Here's how the part is built. I have some questions about the finished solid (model axes, mm). A direction names the side the tool comes from. Coordinates: 2 decimals unless noted, no trailing zeros. Write each loop counter-clockwise with the first axis right and the second up, starting at its lowest first coordinate (ties: lowest second). Pieces come first, ordered by that corner, then holes. Notation, with made-up numbers: (13.25, -3) -> (50.25, -3) arc R27 ccw to (50.25, 34) -> close; hole circle Ø5 at (40, 31.25). An arc over 180 degrees is marked (long way). Use a Markdown table: item, result. Add a question column.
```python
from build123d import *

# Parameters (mm, degrees)
BOSS_EXTRUDE1_DEPTH      = 18
REVOLVE1_ANGLE           = 155
REVOLVE1_OTHER_WAY_ANGLE = 135
CHAMFER1_SIZE            = 2


with BuildPart() as part:
    # Sketch1 → Boss-Extrude1 (new body)
    with BuildSketch(Plane.XY):
        with BuildLine():
            ThreePointArc((26.284248015, 72.215377907), (13.344862454, -75.682475819), (-49.398227804, 58.870515454))
            ThreePointArc((-49.398227804, 58.870515454), (-48.984779038, 59.542460442), (-49.056117508, 60.328183531))
            ThreePointArc((-49.056117508, 60.328183531), (-49.916101751, 61.045004286), (-51.005196829, 60.785626561))
            ThreePointArc((-51.005196829, 60.785626561), (13.778982898, -78.144495202), (27.139298373, 74.564609459))
            ThreePointArc((27.139298373, 74.564609459), (22.507336673, 84.497883381), (32.440610594, 89.129845082))
            ThreePointArc((32.440610594, 89.129845082), (32.488426827, 89.113527981), (32.536863386, 89.099156495))
            ThreePointArc((32.536863386, 89.099156495), (34.05906865, 89.924751911), (33.295660953, 91.479076634))
            ThreePointArc((33.295660953, 91.479076634), (20.158105121, 85.35293374), (26.284248015, 72.215377907))
        make_face()
    extrude(amount=BOSS_EXTRUDE1_DEPTH)

    # Sketch2 → Revolve1 (revolve)
    with BuildSketch(Plane(origin=(0, 0, 0), x_dir=(0, 0, -1), z_dir=(1, 0, 0))):
        Polygon((-14, -74.85), (-16, -76.85), (-2, -76.85), (-4, -74.85), align=None)
    revolve(axis=Axis((0, 0, 0), (0, 0, 1)), revolution_arc=REVOLVE1_ANGLE)

    # Sketch2 → Revolve1 other way (revolve)
    with BuildSketch(Plane(origin=(0, 0, 0), x_dir=(0, 0, -1), z_dir=(1, 0, 0))):
        Polygon((-14, -74.85), (-16, -76.85), (-2, -76.85), (-4, -74.85), align=None)
    revolve(axis=Axis((0, 0, 0), (0, 0, -1)), revolution_arc=REVOLVE1_OTHER_WAY_ANGLE)

    # Chamfer1
    # the kernel refuses this chamfer: 2 mm, written as the material it takes off along each edge
    with BuildSketch(Plane(origin=(31.632976891, 67.83713786, -1.214315162), x_dir=(0.9005003860175051, -0.4348552112856927, 0), z_dir=(0, 0, 1))) as chamfer1_piece_1_section:
        with BuildLine():
            Line((2.027650031, 0), (-CHAMFER1_SIZE * 0.0135447563861, CHAMFER1_SIZE * 0.99990826558))
            Line((-CHAMFER1_SIZE * 0.0135447563861, CHAMFER1_SIZE * 0.99990826558), (0, 0))
            ThreePointArc((0, 0), (1.042503113, 0.006860827), (2.027650031, 0))
        make_face()
    chamfer1_piece_1 = extrude(amount=20.428630325, mode=Mode.PRIVATE)
    chamfer1_piece_1 = chamfer1_piece_1 & Plane(origin=(0, 0, -1.214315162), x_dir=(0.3420201433256637, 0.9396926207859103, 0), z_dir=(0, 0, -1)) * Cylinder(76.85, 49, mode=Mode.PRIVATE)
    add(chamfer1_piece_1, mode=Mode.SUBTRACT)
    with BuildSketch(Plane(origin=(-52.926942572, 52.926942572, -1.214315162), x_dir=(-0.6974643260656699, -0.7166195042459848, 0), z_dir=(0, 0, 1))) as chamfer1_piece_2_section:
        with BuildLine():
            Line((2.027650031, 0), (-CHAMFER1_SIZE * 0.0135447563861, -CHAMFER1_SIZE * 0.99990826558))
            Line((-CHAMFER1_SIZE * 0.0135447563861, -CHAMFER1_SIZE * 0.99990826558), (0, 0))
            ThreePointArc((0, 0), (1.042503113, -0.006860827), (2.027650031, 0))
        make_face()
    chamfer1_piece_2 = extrude(amount=20.428630325, mode=Mode.PRIVATE)
    chamfer1_piece_2 = chamfer1_piece_2 & Plane(origin=(0, 0, -1.214315162), x_dir=(0.3420201433256637, 0.9396926207859103, 0), z_dir=(0, 0, -1)) * Cylinder(76.85, 49, mode=Mode.PRIVATE)
    add(chamfer1_piece_2, mode=Mode.SUBTRACT)


solid = part.part
```
Q1. Suppose I cut it at C-C, the plane z = 8.5. Write out the boundary of the cut face in (x, y), and give its area (3 significant figures).
Q2. Please list where these lines run through material, in increasing order: line 1 (Y direction, x = 28.5, z = 3.25); line 2 (X direction, y = 0, z = 8); line 3 (Y direction, x = 0, z = 8.25).
Q3. Suppose I cut it at A-A, the plane y = 0. Write out the boundary of the cut face in (x, z).
Q4. Will these pins go through, and if not, where does the flat tip stop? pin 1 (8 mm diameter, centred on y = 67.5, z = 5.5, fed in from +X); pin 2 (5 mm diameter, centred on y = -57.5, z = 7.5, fed in from +X); pin 3 (5 mm diameter, centred on x = 2.5, z = 7, fed in from +Y).
Q5. Which directions (+Z, -Z, +X, -X, +Y, -Y) give clear straight access to the entire face, cutting with the end or side of a thin tool? Please do faces 1 (the flat face through (-53, -57, 18)), 2 (the cylindrical face through (63.063, -43.921, 16.291)).
Q6. Thinking about a two-plate mould opening in Y: for faces 3 (the flat face through (-53, -57, 0)), 4 (the conical face through (15.63, -73.33, 14.13)), which applies, released by +Y, released by -Y, zero draft, split by the parting line, or undercut?
Q7. Suppose I cut it at B-B, the plane x = 0. Write out the boundary of the cut face in (y, z).
Answer key:
| question | item | result |
|---|---|---|
| 1 | outline | (-54.34, 51.47) -> (-54.34, 54.34) arc R76.85 cw to (-49.4, 58.87) arc R1.25 ccw to (-51.01, 60.79) arc R79.35 ccw (long way) to (27.14, 74.56) arc R7.75 cw to (32.44, 89.13) arc R1.25 ccw to (33.3, 91.48) arc R10.25 ccw to (26.28, 72.22) arc R76.85 cw to (32.48, 69.65) -> (33.46, 66.96) arc R74.85 cw (long way) to start |
| 1 | area | 1,860 mm^2 |
| 2 | line 1 | y = -74.06 to -70.02, 71.37 to 74.06, 89.49 to 92.02 |
| 2 | line 2 | x = -79.35 to -74.85, 74.85 to 79.35 |
| 2 | line 3 | y = -79.35 to -74.85 |
| 3 | outline | (-79.35, 0) -> (-76.85, 0) -> (-76.85, 2) -> (-74.85, 4) -> (-74.85, 14) -> (-76.85, 16) -> (-76.85, 18) -> (-79.35, 18) -> close; (74.85, 4) -> (76.85, 2) -> (76.85, 0) -> (79.35, 0) -> (79.35, 18) -> (76.85, 18) -> (76.85, 16) -> (74.85, 14) -> close |
| 4 | pin 1 | stops at x = 47.58 |
| 4 | pin 2 | stops at x = 57.2 |
| 4 | pin 3 | stops at y = -74.68 |
| 5 | face 1 | +Z, +X, -X, +Y, -Y |
| 5 | face 2 | none |
| 6 | face 3 | zero draft |
| 6 | face 4 | undercut |
| 7 | outline | (-79.35, 0) -> (-76.85, 0) -> (-76.85, 2) -> (-74.85, 4) -> (-74.85, 14) -> (-76.85, 16) -> (-76.85, 18) -> (-79.35, 18) -> close |
